Input: part model. Units: mm. Frame: model coordinates. A direction names the side the tool comes from. Coordinates: 2 decimals unless noted, no trailing zeros. Order: outer loops, then holes, each group sorted by start corner. A loop starts at its lowest first (then second) coordinate and runs counter-clockwise, first axis right, second up.
from build123d import *

# Parameters (mm, degrees)
SKETCH_1_R      = 4
EXTRUDE_1_DEPTH = 2
SKETCH_2_R      = 1.15
EXTRUDE_2_DEPTH = 5
SKETCH_3_R      = 2.25
EXTRUDE_3_DEPTH = 0.5
SKETCH_4_R      = 2.25
EXTRUDE_4_DEPTH = 1.5
EXTRUDE_4_TAPER = 35


with BuildPart() as part:
    # 스케치1 → 보스-돌출1 (new body)
    with BuildSketch(Plane.XY):
        Circle(SKETCH_1_R)
    extrude(amount=EXTRUDE_1_DEPTH)

    # 스케치2 → 보스-돌출2 (add)
    with BuildSketch(Plane.XY.offset(2)):
        Circle(SKETCH_2_R)
    extrude(amount=EXTRUDE_2_DEPTH)

    # 스케치3 → 보스-돌출3 (add)
    with BuildSketch(Plane.XY.offset(7)):
        Circle(SKETCH_3_R)
    extrude(amount=EXTRUDE_3_DEPTH)

    # 스케치4 → 보스-돌출4 (add)
    with BuildSketch(Plane.XY.offset(7.5)):
        Circle(SKETCH_4_R)
    extrude(amount=EXTRUDE_4_DEPTH, taper=EXTRUDE_4_TAPER)


solid = part.part
Item 1: Cut plane D-D on z = 6.25. Return loops of the section in (x, y), then the cut area to 3 significant figures.
Response values:
outline: circle Ø2.3 at (0, 0)
area: 4.15 mm2
Item 2: Cut plane A-A on y = 0. Return loops of the section in (x, z), then the cut area to 3 significant figures.
Response values:
outline: (-4, 0) - (4, 0) - (4, 2) - (1.15, 2) - (1.15, 7) - (2.25, 7) - (2.25, 7.5) - (1.2, 9) - (-1.2, 9) - (-2.25, 7.5) - (-2.25, 7) - (-1.15, 7) - (-1.15, 2) - (-4, 2) - close
area: 34.9 mm2
Item 3: Access query for faces 5 (the face through (-1, 1, 7)), 6 (the face through (-0.867, -3.905, 0.986)). Directions: +Z, -Z, +X, -X, +Y, -Y. A direction counts if a zero-diameter tool reaches every point of the face in a straight line with its end or side. Return the directions, or none.
Response values:
face 5: none
face 6: +Z, -Z
Item 4: Draft query along Z for faces 1 (the face through (0, 0, 0)), 2 (the face through (0, 0, 9)), 3 (the face through (-0.91, -0.7, 4.46)), 4 (the face through (-0.29, 2.23, 7.25)). Return one class per face: pulls with the +Z half, pulls with the -Z half, needs draft (parallel to the pull), parting line crosses it, or undercut.
Response values:
face 1: pulls with the -Z half
face 2: pulls with the +Z half
face 3: undercut
face 4: needs draft
Item 5: Pin query (flat end, axial travel): pin 1 Ø1.5 at (x, z) = (3, 5.5) entering from +Y; pin 2 Ø1.5 at (y, z) = (1, 3.5) entering from -X; pin 3 Ø1 at (y, z) = (-0.5, 8) entering from +X. Return the tip coordinate at first contact, or that it passes through.
Response values:
pin 1: passes through
pin 2: stops at x = -1.12
pin 3: stops at x = 2.21
Item 6: Ray query, probe 1 along Z at (x, y) = (1.5, 3); probe 2 along Y at (x, z) = (0, 5); probe 3 along Y at (x, z) = (2.75, 1). Return the intervals inside material, ascending.
Response values:
probe 1: z = 0 to 2
probe 2: y = -1.15 to 1.15
probe 3: y = -2.9 to 2.9
Item 7: Cut plane C-C on z = 0.5. Return loops of the section in (x, y).
Response values:
outline: circle Ø8 at (0, 0)
